Work out the finished part from the listing and answer in its coordinate system (mm). Face numbers are marked on the shaded views. Round coordinates to 2 decimals unless told otherwise and drop trailing zeros. Order: outer loops, then holes, each group sorted by start corner. A loop starts at its lowest first (then second) coordinate and runs counter-clockwise, first axis right, second up. Notation, with made-up numbers: (0, 53) - (58, 53) arc R27 cw to (58, 80) - close; hole circle Ø10 at (-18.5, -19). An arc over 180 degrees is marked (long way). Put each result on its own line as item: value.
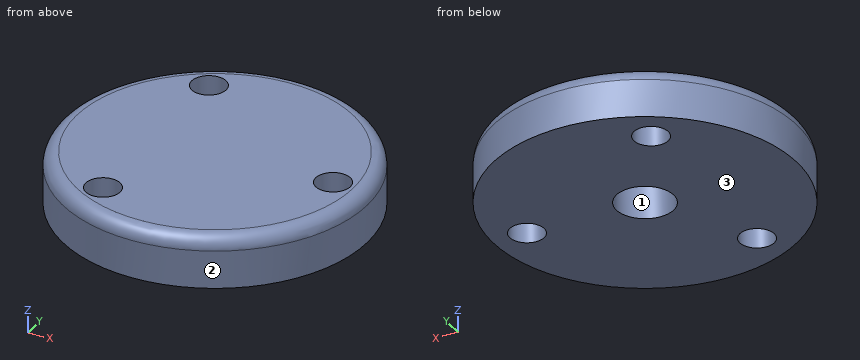
Autodesk Inventor part; units mm, degrees
ref_plane "YZ Plane" through (0, 0, 0) normal (1, 0, 0) x (0, 1, 0)
ref_plane "XZ Plane" through (0, 0, 0) normal (0, 1, 0) x (-1, 0, 0)
ref_plane "XY Plane" through (0, 0, 0) normal (0, 0, 1) x (1, 0, 0)
sketch "Sketch1" plane through (0, 0, 0) normal (0, 0, 1) x (1, 0, 0)
  circle A0 centre (0, 0) radius 22
  circle A1 centre (17, 0) radius 2.5
  circle A2 centre (-8.5, 14.7224) radius 2.5
  circle A3 centre (-8.5, -14.7224) radius 2.5
  dimension "d0" = 44
  dimension "d1" = 5
  dimension "d2" = 17
  dimension "d5" = 360
extrude "Extrusion1" add sketch "Sketch1" along normal blind 7.5
fillet "Fillet1" radius 2 1 edges at (-22, 0, 7.5)
sketch "Sketch2" plane through (0, 0, 0) normal (0, 0, -1) x (-1, 0, 0)
  circle A0 centre (0, 0) radius 4.15
  dimension "d10" = 8.3
extrude "Extrusion2" cut sketch "Sketch2" against normal blind 5
properties part number "AA014" material "ABS Plastic"
1) A cutting plane is placed at C-C on x = -9. Give the number of separate pieces and of enclosed holes in the cut face, then the cut area to 3 significant figures.
Findings below:
separate pieces: 3
enclosed holes: 0
area: 226 mm2
2) A cutting plane is placed at D-D on z = 6.25. Write down the section's boundary in (x, y).
Findings below:
outline: circle Ø43.71 at (0, 0); hole circle Ø5 at (-8.5, -14.72); hole circle Ø5 at (-8.5, 14.72); hole circle Ø5 at (17, 0)
3) A cutting plane is placed at B-B on x = 0. Write down the section's boundary in (y, z), then the cut area to 3 significant figures.
Findings below:
outline: (-22, 0) - (-4.15, 0) - (-4.15, 5) - (4.15, 5) - (4.15, 0) - (22, 0) - (22, 5.5) arc R2 ccw to (20, 7.5) - (-20, 7.5) arc R2 ccw to (-22, 5.5) - close
area: 287 mm2
4) Given pin 1 Ø6.5 at (x, y) = (17, 0) entering from +Z; pin 2 Ø7.5 at (x, y) = (0, 0) entering from -Z; pin 3 Ø1.5 at (y, z) = (-12, 3.5) entering from -X; pin 4 Ø2 at (y, z) = (13.5, 6.5) entering from +X, each flat-ended and moving along its own axis, determine where each tip first touches the part or whether it passes through.
Findings below:
pin 1: stops at z = 7.5
pin 2: stops at z = 5
pin 3: stops at x = -18.91
pin 4: stops at x = 17.94
5) A cutting plane is placed at A-A on y = 0. Write down the section's boundary in (x, z).
Findings below:
outline: (-22, 0) - (-4.15, 0) - (-4.15, 5) - (4.15, 5) - (4.15, 0) - (14.5, 0) - (14.5, 7.5) - (-20, 7.5) arc R2 ccw to (-22, 5.5) - close; (19.5, 0) - (22, 0) - (22, 5.5) arc R2 ccw to (20, 7.5) - (19.5, 7.5) - close
6) Straight lines are drawn through the part: L1, parallel to Y at x = 0, z = 1.65; L2, parallel to Y at x = -8, z = 1; L3, parallel to Y at x = -8.5, z = 3.5. For each, find the intervals that lie inside material, in ascending order. Write a range as from..to.
Findings below:
L1: y = -22..-4.15, 4.15..22
L2: y = -20.49..-17.17, -12.27..12.27, 17.17..20.49
L3: y = -20.29..-17.22, -12.22..12.22, 17.22..20.29
7) For a pull along X with two mould halves and no side action, classify the marked faces 1, 2 and 3 as pulls with the +X half, pulls with the -X half, needs draft (parallel to the pull), parting line crosses it, or undercut.
Findings below:
face 1: undercut
face 2: parting line crosses it
face 3: needs draft
